from build123d import *

# Parameters (mm, degrees)
BOSS_EXTRUDE1_DEPTH = 35
FILLET1_R           = 4
FILLET2_R           = 4


with BuildPart() as part:
    # Sketch1 → Boss-Extrude1 (new body)
    with BuildSketch(Plane(origin=(0, 0, 0), x_dir=(1, 0, 0), z_dir=(0, 1, 0))):
        with BuildLine():
            Line((-45.961922075, 19.685063351), (-47.800398958, 20.472465885))
            ThreePointArc((-47.800398958, 20.472465885), (-46.25587256, 23.756983262), (-44.4859922, 26.925759005))
            Line((-44.4859922, 26.925759005), (-47.05249175, 28.479168178))
            ThreePointArc((-47.05249175, 28.479168178), (-55, 0), (-47.05249175, -28.479168178))
            Line((-47.05249175, -28.479168178), (-44.4859922, -26.925759005))
            ThreePointArc((-44.4859922, -26.925759005), (-46.25587256, -23.756983262), (-47.800398958, -20.472465885))
            Line((-47.800398958, -20.472465885), (-45.961922075, -19.685063351))
            ThreePointArc((-45.961922075, -19.685063351), (-50, 0), (-45.961922075, 19.685063351))
        make_face()
    extrude(amount=BOSS_EXTRUDE1_DEPTH)

    # Fillet1
    fillet1_edges = [part.edges().sort_by_distance(p)[0] for p in [
        (-46.881160517, 0, -20.078764618),
        (-46.881160517, 0, 20.078764618),
        (-46.881160517, 35, 20.078764618),
        (-46.881160517, 35, -20.078764618),
    ]]
    fillet(fillet1_edges, radius=FILLET1_R)

    # Fillet2
    fillet2_edges = [part.edges().sort_by_distance(p)[0] for p in [
        (-45.769241975, 0, 27.702463591),
        (-45.769241975, 0, -27.702463591),
        (-45.769241975, 35, 27.702463591),
        (-45.769241975, 35, -27.702463591),
    ]]
    fillet(fillet2_edges, radius=FILLET2_R)


solid = part.part
Design review of the part built by this model. Coordinates are the model's own, in mm. A direction names the side the tool comes from. Round coordinates to 2 decimals unless told otherwise and drop trailing zeros. Write each loop counter-clockwise with the first axis right and the second up, starting at its lowest first coordinate (ties: lowest second). Pieces come first, ordered by that corner, then holes. Notation, with made-up numbers: M 11.5,-3 L 47.5,-3 A23 cw 47.5,16 Z; hole C -17.5,24 d3. An arc over 180 degrees is marked long. One line per item, written item: value. Start each with the question number.
1. Draft analysis for pull direction Z (two halves, no side actions). For faces 5 (the face through (-46.31, 1.14, 26.62)), 6 (the face through (-55, 17, 0)), 7 (the face through (-46.629, 17.255, -23.016)), state which applies: pulls with the +Z half, pulls with the -Z half, needs draft (parallel to the pull), parting line crosses it, or undercut.
2. Take a section at B-B on z = -14.5. State the section outline as (x, y) points, then the cut area to 3 significant figures.
3. For faces 1 (the face through (-46.894, 17.311, 20.084)), 2 (the face through (-47.27, 1.2, -19)), 3 (the face through (-47.24, 33.8, 18.99)), 4 (the face through (-51, 35, 0)), list the 3-axis set-ups (+Z, -Z, +X, -X, +Y, -Y) from which the entire face can be reached by the end or side of a thin tool; tool diameter is ignored.
4. Take a section at C-C on y = 32. State the section outline as (x, z) points.
5. Clearance check with flat-ended pins moving along their axes: P1, Ø8, axis at y = 7.5, z = -16.5, coming from the -X side; P2, Ø6, axis at x = -46, y = 11.5, coming from the +Z side; P3, Ø5, axis at y = 16.5, z = 11, coming from the +X side. State where each tip first meets the part, or that it passes through.
6. To check wall thickness, follow probe 1 along Z at (x, y) = (-50.25, 14.5); probe 2 along X at (y, z) = (14, -22); probe 3 along X at (y, z) = (8.5, 25). State the ranges of each line that lie inside material, in increasing order. Write a range as from..to.
7. Take a section at D-D on x = -53.25. State the section outline as (y, z) points.
8. Take a section at A-A on y = 28. State the section outline as (x, z) points.
Computed:
1. face 5: pulls with the +Z half
1. face 6: parting line crosses it
1. face 7: undercut
2. outline: M -53.05,0 L -47.85,0 L -47.85,35 L -53.05,35 Z
2. area: 182 mm²
3. face 1: +X, +Y, -Y
3. face 2: +X, -Y
3. face 3: +X, +Y
3. face 4: +Z, -Z, +X, -X, +Y
4. outline: M -47.85,-20.36 L -46.01,-19.57 A50 cw -46.01,19.57 L -47.85,20.36 A52 cw -44.55,26.82 L -47.12,28.37 A55 ccw -47.12,-28.37 L -44.55,-26.82 A52 cw Z
5. P1: stops at x = -53.56
5. P2: stops at z = 28.48
5. P3: stops at x = -48.14
6. probe 1: z = -22.36..22.36
6. probe 2: x = -50.41..-47.12
6. probe 3: x = -48.99..-45.6
7. outline: M 0,-13.76 L 35,-13.76 L 35,13.76 L 0,13.76 Z
8. outline: M -47.8,-20.47 L -45.96,-19.69 A50 cw -45.96,19.69 L -47.8,20.47 A52 cw -44.49,26.93 L -47.05,28.48 A55 ccw -47.05,-28.48 L -44.49,-26.93 A52 cw Z
